Source: CAD feature listing. Evaluate the final solid. Frame: model axes, mm. Coordinates: 2 decimals unless noted, no trailing zeros. Write each loop counter-clockwise with the first axis right and the second up, starting at its lowest first coordinate (ties: lowest second). Pieces come first, ordered by that corner, then holes. Notation, with made-up numbers: M 1.25,-29 L 23.25,-29 A31 ccw 23.25,-2 Z; hole C -26,51.25 d9. An arc over 180 degrees is marked long. Write item = value, one per line. Start each with the question number.
1. Line query: line 1 along X through (y, z) = (1.7, -84); line 2 along Z through (x, y) = (-28, 0.25); line 3 along X through (y, z) = (1.8, 86). Output: solid intervals per line, ascending.
2. Section query A-A (y = 0.95). Give the number of separate pieces and of enclosed holes in the cut face, then the cut area to 3 significant figures.
3. Section query B-B (x = -13.5). Output: boundary loops of the cut face in (y, z).
4. Pull-direction query (X, two-part tool) for faces 1 (the face through (-55.2, 1.5, -82.3)), 2 (the face through (55.2, 1.5, -82.3)), 3 (the face through (4.19, 1.48, 0.01)); classes: pulls with the +X half, pulls with the -X half, needs draft (parallel to the pull), parting line crosses it, or undercut.
5. Pin query (flat end, axial travel): pin 1 Ø1.5 at (y, z) = (1, -93.5) entering from +X. Return the tip coordinate at first contact, or that it passes through.
```python
from build123d import *

# Parameters (mm, degrees)
SKETCH2_W           = 135
SKETCH2_H           = 190
BOSS_EXTRUDE2_DEPTH = 3
SKETCH3_R           = 1.75
CUT_EXTRUDE1_DEPTH  = 117.577227622
FILLET1_SIZE        = 12.5
FILLET1_SIZE_2      = 50
FILLET2_SIZE        = 12.5
FILLET2_SIZE_2      = 50
CHAMFER2_SIZE       = 25
CHAMFER3_SIZE       = 25
CUT_EXTRUDE5_DEPTH  = 117.577227764
SKETCH8_R           = 1.75
CUT_EXTRUDE6_DEPTH  = 117.577227764
SKETCH11_R          = 1.75
CUT_EXTRUDE8_DEPTH  = 117.577227764
SKETCH12_R          = 1.75
CUT_EXTRUDE9_DEPTH  = 117.577227764
SKETCH18_R          = 1.75
CUT_EXTRUDE10_DEPTH = 117.577227764
SKETCH19_R          = 1.75
CUT_EXTRUDE11_DEPTH = 117.577227764
SKETCH20_R          = 1.75
CUT_EXTRUDE12_DEPTH = 10


with BuildPart() as part:
    # Sketch2 → Boss-Extrude2 (new body)
    with BuildSketch(Plane(origin=(0, 0, 0), x_dir=(1, 0, 0), z_dir=(0, 1, 0))):
        Rectangle(SKETCH2_W, SKETCH2_H)
    extrude(amount=BOSS_EXTRUDE2_DEPTH)

    # Sketch3 → Cut-Extrude1 (cut, through all)
    with BuildSketch(Plane(origin=(0, 3, 0), x_dir=(1, 0, 0), z_dir=(0, 1, 0))):
        with Locations(Location((-27.5, -50, 0), (0, 0, 270))):
            Circle(SKETCH3_R)
        with Locations(Location((27.5, -50, 0), (0, 0, 90))):
            Circle(SKETCH3_R)
        with Locations(Location((-50, -85, 0), (0, 0, 270))):
            Circle(SKETCH3_R)
        with Locations(Location((50, -85, 0), (0, 0, 90))):
            Circle(SKETCH3_R)
    extrude(amount=-CUT_EXTRUDE1_DEPTH, mode=Mode.SUBTRACT)

    # Fillet1
    # an asymmetric fillet: 50, 12.5 mm, written as the material it takes off along each edge
    with BuildSketch(Plane(origin=(-67.5, -125, 95), x_dir=(0, 0, -1), z_dir=(0, 1, 0))) as fillet1_piece_1:
        with BuildLine():
            Bezier((FILLET1_SIZE, 0), (0, 0), (0, -FILLET1_SIZE_2), weights=[1, 0.707106781, 1])
            Line((0, -FILLET1_SIZE_2), (0, 0))
            Line((0, 0), (FILLET1_SIZE, 0))
        make_face()
    extrude(amount=253, mode=Mode.SUBTRACT)

    # Fillet2
    # an asymmetric fillet: 50, 12.5 mm, written as the material it takes off along each edge
    with BuildSketch(Plane(origin=(67.5, -125, 95), x_dir=(0, 0, -1), z_dir=(0, 1, 0))) as fillet2_piece_1:
        with BuildLine():
            Bezier((FILLET2_SIZE, 0), (0, 0), (0, FILLET2_SIZE_2), weights=[1, 0.707106781, 1])
            Line((0, FILLET2_SIZE_2), (0, 0))
            Line((0, 0), (FILLET2_SIZE, 0))
        make_face()
    extrude(amount=253, mode=Mode.SUBTRACT)

    # Chamfer2
    chamfer2_edges = [part.edges().sort_by_distance(p)[0] for p in [
        (67.5, 1.5, -95),
    ]]
    chamfer(chamfer2_edges, length=CHAMFER2_SIZE)

    # Chamfer3
    chamfer3_edges = [part.edges().sort_by_distance(p)[0] for p in [
        (-67.5, 1.5, -95),
    ]]
    chamfer(chamfer3_edges, length=CHAMFER3_SIZE)

    # Sketch7 → Cut-Extrude5 (cut, through all)
    with BuildSketch(Plane(origin=(0, 3, 0), x_dir=(1, 0, 0), z_dir=(0, 1, 0))):
        with BuildLine():
            Line((24, 91.5), (24, 95))
            Line((24, 95), (-24, 95))
            Line((-24, 95), (-24, 91.5))
            ThreePointArc((-24, 91.5), (0, 67.5), (24, 91.5))
        make_face()
    extrude(amount=-CUT_EXTRUDE5_DEPTH, mode=Mode.SUBTRACT)

    # Sketch8 → Cut-Extrude6 (cut, through all)
    with BuildSketch(Plane(origin=(0, 3, 0), x_dir=(1, 0, 0), z_dir=(0, 1, 0))):
        with Locations(Location((-27, 91.5, 0), (0, 0, 270))):
            Circle(SKETCH8_R)
        with Locations(Location((27, 91.5, 0), (0, 0, 270))):
            Circle(SKETCH8_R)
    extrude(amount=-CUT_EXTRUDE6_DEPTH, mode=Mode.SUBTRACT)

    # Sketch11 → Cut-Extrude8 (cut, through all)
    with BuildSketch(Plane(origin=(0, 3, 0), x_dir=(1, 0, 0), z_dir=(0, 1, 0))):
        with Locations(Location((47.347456736, 85.202795796, 0), (0, 0, 270))):
            Circle(SKETCH11_R)
        with Locations(Location((64, 65, 0), (0, 0, 270))):
            Circle(SKETCH11_R)
        with Locations(Location((-64, 65, 0), (0, 0, 270))):
            Circle(SKETCH11_R)
        with Locations(Location((-47.347456736, 85.202795796, 0), (0, 0, 270))):
            Circle(SKETCH11_R)
    extrude(amount=-CUT_EXTRUDE8_DEPTH, mode=Mode.SUBTRACT)

    # Sketch12 → Cut-Extrude9 (cut, through all)
    with BuildSketch(Plane(origin=(0, 0, 0), x_dir=(-1, 0, 0), z_dir=(0, -1, 0))):
        with Locations(Location((45, -33, 0), (0, 0, 90))):
            Circle(SKETCH12_R)
        with Locations(Location((-5.9, -26.63, 0), (0, 0, 90))):
            Circle(SKETCH12_R)
        with Locations(Location((45, 15.6, 0), (0, 0, 90))):
            Circle(SKETCH12_R)
        with Locations(Location((-5.9, 0.37, 0), (0, 0, 90))):
            Circle(SKETCH12_R)
    extrude(amount=-CUT_EXTRUDE9_DEPTH, mode=Mode.SUBTRACT)

    # Sketch18 → Cut-Extrude10 (cut, through all)
    with BuildSketch(Plane(origin=(0, 3, 0), x_dir=(1, 0, 0), z_dir=(0, 1, 0))):
        with Locations(Location((20.83, -28.2, 0), (0, 0, 270))):
            Circle(SKETCH18_R)
        with Locations(Location((20.83, 11.3, 0), (0, 0, 270))):
            Circle(SKETCH18_R)
        with Locations(Location((60.33, 11.3, 0), (0, 0, 270))):
            Circle(SKETCH18_R)
        with Locations(Location((60.33, -28.2, 0), (0, 0, 270))):
            Circle(SKETCH18_R)
    extrude(amount=-CUT_EXTRUDE10_DEPTH, mode=Mode.SUBTRACT)

    # Sketch19 → Cut-Extrude11 (cut, through all)
    with BuildSketch(Plane(origin=(0, 3, 0), x_dir=(1, 0, 0), z_dir=(0, 1, 0))):
        with Locations(Location((57.5, 50.8, 0), (0, 0, 270))):
            Circle(SKETCH19_R)
        with Locations(Location((-57.5, 27.8, 0), (0, 0, 270))):
            Circle(SKETCH19_R)
    extrude(amount=-CUT_EXTRUDE11_DEPTH, mode=Mode.SUBTRACT)

    # Sketch20 → Cut-Extrude12 (cut)
    with BuildSketch(Plane(origin=(0, 0, 0), x_dir=(-1, 0, 0), z_dir=(0, -1, 0))):
        with Locations(Location((19.5, 69.019658785, 0), (0, 0, 90))):
            Circle(SKETCH20_R)
        with Locations(Location((-19.5, 69.019658785, 0), (0, 0, 90))):
            Circle(SKETCH20_R)
    extrude(amount=-CUT_EXTRUDE12_DEPTH, mode=Mode.SUBTRACT)


solid = part.part
```
Results are:
q1.line_1 = -53.5 to -48.62, -46.08 to -22.8, 22.8 to 46.08, 48.62 to 53.5
q1.line_2 = -95 to -92.94, -90.06 to 48.32, 51.68 to 94.72
q1.line_3 = -65.5 to -51.44, -48.56 to 48.56, 51.44 to 65.5
q2.separate_pieces = 1
q2.enclosed_holes = 22
q2.area = 23,500 mm^2
q3.outline = M 0,-71.66 L 3,-71.66 L 3,95 L 0,95 Z
q4.face_1 = pulls with the -X half
q4.face_2 = pulls with the +X half
q4.face_3 = undercut
q5.pin_1 = 44.75
